```python
from build123d import *

# Parameters (mm, degrees)
F0_W     = 81.6
F0_H     = 35.75
F0_R     = 1
F0_R_2   = 6.65
F1_DEPTH = 2
F2_DEPTH = 64.3
F3_R     = 6.65
F3_R_2   = 1
F4_DEPTH = 81.601


with BuildPart() as f1:
    # F0 (on Top) → F1 (new body)
    with BuildSketch(Plane.XY):
        Rectangle(F0_W, F0_H)
        Polygon((-38.8, -15.875), (-38.8, 15.875), (0, 15.875), (38.8, 15.875), (38.8, -15.875), (0, -15.875), align=None, mode=Mode.SUBTRACT)
        Polygon((0, 15.875), (-38.8, 15.875), (-38.8, -15.875), (0, -15.875), (38.8, -15.875), (38.8, 15.875), align=None)
        with Locations((-35.5, -8.425)):
            Circle(F0_R, mode=Mode.SUBTRACT)
        with Locations((-25, -8.425)):
            Circle(F0_R_2, mode=Mode.SUBTRACT)
        with Locations((-14.5, -8.425)):
            Circle(F0_R, mode=Mode.SUBTRACT)
        with Locations((14.5, -8.425)):
            Circle(F0_R, mode=Mode.SUBTRACT)
        with Locations((25, -8.425)):
            Circle(F0_R_2, mode=Mode.SUBTRACT)
        with Locations((35.5, -8.425)):
            Circle(F0_R, mode=Mode.SUBTRACT)
        with Locations((-35.5, 12.575)):
            Circle(F0_R, mode=Mode.SUBTRACT)
        with Locations((-14.5, 12.575)):
            Circle(F0_R, mode=Mode.SUBTRACT)
        with Locations((14.5, 12.575)):
            Circle(F0_R, mode=Mode.SUBTRACT)
        with Locations((35.5, 12.575)):
            Circle(F0_R, mode=Mode.SUBTRACT)
    extrude(amount=F1_DEPTH)

    # F0 (on Top) → F2 (join)
    with BuildSketch(Plane.XY):
        Rectangle(F0_W, F0_H)
        Polygon((-38.8, -15.875), (-38.8, 15.875), (0, 15.875), (38.8, 15.875), (38.8, -15.875), (0, -15.875), align=None, mode=Mode.SUBTRACT)
    extrude(amount=F2_DEPTH)

    # F3 (on face) → F4 (cut, through all)
    with BuildSketch(Plane.YZ.offset(40.8)):
        with Locations((-7.925, 51)):
            Circle(F3_R)
        with Locations((-7.925, 61.5)):
            Circle(F3_R_2)
        with Locations((-7.925, 40.5)):
            Circle(F3_R_2)
        with Locations((13.075, 40.5)):
            Circle(F3_R_2)
        with Locations((13.075, 61.5)):
            Circle(F3_R_2)
    extrude(amount=-F4_DEPTH, mode=Mode.SUBTRACT)


solid = f1.part
```
Build history of the part. All positions in model axes, mm. A direction names the side the tool comes from. Coordinates: 2 decimals unless noted, no trailing zeros. Order: outer loops, then holes, each group sorted by start corner. A loop starts at its lowest first (then second) coordinate and runs counter-clockwise, first axis right, second up.
Item 1: Drill centre lines: L1, parallel to Y at x = 14, z = 46.5 (3 decimals); L2, parallel to X at y = -11.5, z = 14; L3, parallel to Y at x = -35.5, z = 0.9 (3 decimals). Where is each one in solid material? Low to high.
Filled in:
L1: y = -17.875 to -15.875, 15.875 to 17.875
L2: x = -40.8 to -38.8, 38.8 to 40.8
L3: y = -17.875 to -9.425, -7.425 to 11.575, 13.575 to 17.875
Item 2: Tool access for faces 1 (the flat face through (40.8, 0, 32)), 2 (the flat face through (-1, 0, 2)): list every direction of +Z, -Z, +X, -X, +Y, -Y with a clear straight run to the whole face (end or side of a thin tool).
Filled in:
face 1: +Z, -Z, +X, +Y, -Y
face 2: +Z
Item 3: Saw through at D-D on z = 51. List the corners of the cut face in (x, y) (3 decimals), then the cut area to 3 significant figures.
Filled in:
outline: (-40.8, -17.875) - (40.8, -17.875) - (40.8, -14.575) - (38.8, -14.575) - (38.8, -15.875) - (-38.8, -15.875) - (-38.8, -14.575) - (-40.8, -14.575) - close; (-40.8, -1.275) - (-38.8, -1.275) - (-38.8, 15.875) - (38.8, 15.875) - (38.8, -1.275) - (40.8, -1.275) - (40.8, 17.875) - (-40.8, 17.875) - close
area: 400 mm2
Item 4: Saw through at C-C on z = 18. List the corners of the cut face in (x, y) (3 decimals), then the cut area to 3 significant figures.
Filled in:
outline: (-40.8, -17.875) - (40.8, -17.875) - (40.8, 17.875) - (-40.8, 17.875) - close; hole (-38.8, -15.875) - (38.8, -15.875) - (38.8, 15.875) - (-38.8, 15.875) - close
area: 453 mm2
Item 5: Drop a flat-ended pin along its axis: pin 1 Ø5 at (x, y) = (-16, -1) entering from +Z. Give the stop position or say it passes through.
Filled in:
pin 1: stops at z = 2
Item 6: Mould opens along Y. For faces 3 (the flat face through (1, -15.875, 33)), 4 (the flat face through (-1, 17.875, 32)), 5 (the cylindrical face through (-31.644, -8.133, 0.986)), 6 (the flat face through (-1, 0, 0)) say: released by +Y, released by -Y, zero draft, split by the parting line, or undercut.
Filled in:
face 3: undercut
face 4: released by +Y
face 5: undercut
face 6: zero draft
Item 7: Saw through at A-A on x = 14.5. List the corners of the cut face in (y, z) (3 decimals).
Filled in:
outline: (-17.875, 0) - (-9.425, 0) - (-9.425, 2) - (-15.875, 2) - (-15.875, 64.3) - (-17.875, 64.3) - close; (-7.425, 0) - (11.575, 0) - (11.575, 2) - (-7.425, 2) - close; (13.575, 0) - (17.875, 0) - (17.875, 64.3) - (15.875, 64.3) - (15.875, 2) - (13.575, 2) - close
Item 8: Saw through at B-B on x = -25. List the corners of the cut face in (y, z) (3 decimals), then the cut area to 3 significant figures.
Filled in:
outline: (-17.875, 0) - (-15.075, 0) - (-15.075, 2) - (-15.875, 2) - (-15.875, 64.3) - (-17.875, 64.3) - close; (-1.775, 0) - (17.875, 0) - (17.875, 64.3) - (15.875, 64.3) - (15.875, 2) - (-1.775, 2) - close
area: 294 mm2
